Check sheet for the modelled part. Datum: model origin and axes. Units: mm. Face numbers are marked on the shaded views. Round coordinates to 2 decimals unless told otherwise and drop trailing zeros. Order: outer loops, then holes, each group sorted by start corner. A loop starts at its lowest first (then second) coordinate and runs counter-clockwise, first axis right, second up.
Q1. Cross-section at A-A on x = 7. Record the cut outline in (y, z).
Q2. Mould release check, pull along Y, two halves, no side actions. Record for the marked faces 1, 2 and 3: +Y half, -Y half, draft (parallel to the pull), parting line (faces both ways), or undercut.
Q3. Cross-section at C-C on z = -91.5. Record the cut outline in (x, y), then the cut area to 3 significant figures.
Q4. Depth check by flat-ended pin: P1, Ø4, axis at x = 100.5, y = 162, coming from the -Z side; P2, Ø11, axis at x = -104.5, y = 172, coming from the +Z side. Enter the tip coordinate at first touch or a pass-through.
Q5. Cross-section at B-B on y = 288.5. Record the cut outline in (x, z).
Q6. Cross-section at D-D on z = 0. Record the cut outline in (x, y), then the cut area to 3 significant figures.
Q7. Scan lines: probe 1 along Z at (x, y) = (154, 102.5); probe 2 along X at (y, z) = (159.5, 34); probe 3 along Y at (x, z) = (-168.5, -90.5). Record each from-to range of solid material in increasing order.
Autodesk Inventor part; units mm, degrees
ref_plane "YZ Plane" through (0, 0, 0) normal (1, 0, 0) x (0, 1, 0)
ref_plane "XZ Plane" through (0, 0, 0) normal (0, 1, 0) x (-1, 0, 0)
ref_plane "XY Plane" through (0, 0, 0) normal (0, 0, 1) x (1, 0, 0)
sketch "Boceto1" plane through (0, 0, 0) normal (0, 1, 0) x (-1, 0, 0)
  line L0 (200, 200) -> (-200, 200)
  line L1 (-200, 200) -> (-200, -200)
  line L2 (-200, -200) -> (200, -200)
  line L3 (200, -200) -> (200, 200)
  point P0 (0, 0)
  dimension "d0" = 400
  dimension "L" = 400
  dimension "d2" = 200
  dimension "d3" = 200
extrude "Extrusión1" add sketch "Boceto1" along normal blind 150
sketch "Boceto3" plane through (0, 150, 0) normal (0, 1, 0) x (1, 0, 0)
  circle A0 centre (0, -121) radius 39
  line L0 (200, 200) -> (-200, 200)
  line L1 (-200, -200) -> (200, -200)
  point P0 (0, 0)
  dimension "D" = 78
  dimension "d27" = 79
extrude "Extrusión2" [suppressed]
ref_plane "Plano de trabajo1" through (0, 0, 200) normal (1, 0, 0) x (0, 0, -1)
ref_plane "Plano de trabajo2" through (-200, 0, 0) normal (0, 0, 1) x (1, 0, 0)
sketch "Boceto4" plane through (0, 150, 0) normal (0, 1, 0) x (1, 0, 0)
  line L0 (-97.5, 140) -> (-97.5, -140)
  line L1 (97.5, 140) -> (97.5, -140)
  line L2 (200, 200) -> (-200, 200)
  circle A0 centre (0, -121) radius 39
  line L3 (-200, -200) -> (200, -200)
  line L4 (-97.5, -140) -> (-107.5, -140)
  line L5 (-107.5, -140) -> (-107.5, 140)
  line L6 (-107.5, 140) -> (-97.5, 140)
  line L7 (-97.5, 140) -> (-97.5, -140)
  line L8 (97.5, -140) -> (107.5, -140)
  line L9 (107.5, -140) -> (107.5, 140)
  line L10 (107.5, 140) -> (97.5, 140)
  line L11 (97.5, 140) -> (97.5, -140)
  point P0 (0, 0)
  dimension "Lriel" = 280
  dimension "d13" = 60
  dimension "d14" = 280
  dimension "d15" = 60
  dimension "d19" = 10
  dimension "d20" = 280
  dimension "d21" = 97.5
  dimension "d22" = 10
  dimension "d23" = 280
  dimension "d24" = 97.5
extrude "Extrusión3" add sketch "Boceto4" along normal blind 38 contours L0 L4 L5 L6 | L10 L9 L8 L1
sketch "Boceto5" plane through (0, 150, 0) normal (0, 1, 0) x (1, 0, 0)
  line L0 (-200, 200) -> (-200, -200)
  line L1 (-200, 200) -> (-200, 175)
  line L2 (-200, 175.482) -> (-195, 175.482)
  line L3 (-195, 175.482) -> (-195, 195.482)
  line L4 (-195, 195.482) -> (-175, 195.482)
  line L5 (-175, 195.482) -> (-175, 200)
  line L6 (200, 200) -> (-200, 200)
  line L7 (-200, 200) -> (-175, 200)
  line L8 (-200, -200) -> (-200, -175)
  line L9 (-200, -175) -> (-195, -175)
  line L10 (-195, -175) -> (-195, -195)
  line L11 (-195, -195) -> (-175, -195)
  line L12 (-175, -195) -> (-175, -200)
  line L13 (-200, -200) -> (200, -200)
  line L14 (-175, -200) -> (-200, -200)
  line L15 (200, -200) -> (200, 200)
  line L16 (200, -200) -> (200, -175)
  line L17 (200, -175) -> (195, -175)
  line L18 (195, -175) -> (195, -195)
  line L19 (195, -195) -> (175, -195)
  line L20 (175, -195) -> (175, -200)
  line L21 (200, -200) -> (175, -200)
  line L22 (200, 200) -> (200, 175)
  line L23 (200, 175) -> (195, 175)
  line L24 (195, 175) -> (195, 195)
  line L25 (195, 195) -> (175, 195)
  line L26 (175, 195) -> (175, 200)
  line L27 (200, 200) -> (175, 200)
  point P0 (0, 0)
  dimension "d28" = 25
  dimension "d29" = 5
  dimension "d30" = 20
  dimension "d31" = 20
  dimension "d32" = 25
  dimension "d33" = 5
  dimension "d34" = 20
  dimension "d35" = 20
  dimension "d36" = 25
  dimension "d37" = 5
  dimension "d38" = 20
  dimension "d39" = 20
  dimension "d40" = 25
  dimension "d41" = 5
  dimension "d42" = 20
  dimension "d43" = 20
extrude "Extrusión4" add sketch "Boceto5" along normal blind 200 contours L6 L5 L4 L3 L2 L0 | L6 L15 L23 L24 L25 L26 | L9 L10 L11 L12 L13 L0 | L15 L13 L20 L19 L18 L17
sketch "Boceto6" plane through (0, 350, 0) normal (0, 1, 0) x (1, 0, 0)
  line L0 (-200, 200) -> (-200, -200)
  line L1 (-200, -200) -> (200, -200)
  line L2 (200, -200) -> (200, 200)
  line L3 (200, 200) -> (-200, 200)
  line L4 (-200, 200) -> (-200, -200)
  point P0 (0, 0)
extrude "Extrusión5" add sketch "Boceto6" along normal blind 5
sketch "Boceto7" plane through (0, 150, 0) normal (0, 1, 0) x (1, 0, 0)
  line L0 (-200, 200) -> (-200, -200)
  line L1 (200, 200) -> (-200, 200)
  line L2 (200, -200) -> (200, 200)
  line L3 (-200, -200) -> (200, -200)
  circle A0 centre (154, 0) radius 39
  point P0 (0, 0)
  dimension "d48" = 78
  dimension "d49" = 200
  dimension "d50" = 46
extrude "Extrusión6" cut sketch "Boceto7" against normal blind 200.5 contours A0
sketch "Boceto8" plane through (107.5, 150, 140) normal (1, 0, 0) x (0, 0, -1)
  line L0 (61.75, 6.3333) -> (78.25, 6.3333) construction
  line L1 (61.75, 10.3333) -> (78.25, 10.3333)
  line L2 (78.25, 2.3333) -> (61.75, 2.3333)
  arc A0 (61.75, 10.3333) -> (61.75, 2.3333) centre (61.75, 6.3333) ccw
  arc A1 (78.25, 2.3333) -> (78.25, 10.3333) centre (78.25, 6.3333) ccw
  line L3 (0, 38) -> (280, 38)
  line L4 (0, 0) -> (0, 38)
  line L5 (198.75, 6.3333) -> (221.25, 6.3333) construction
  line L6 (315.482, 0) -> (-35, 0)
  line L7 (198.75, 10.3333) -> (221.25, 10.3333)
  line L8 (221.25, 2.3333) -> (198.75, 2.3333)
  arc A2 (198.75, 10.3333) -> (198.75, 2.3333) centre (198.75, 6.3333) ccw
  arc A3 (221.25, 2.3333) -> (221.25, 10.3333) centre (221.25, 6.3333) ccw
  line L9 (280, 0) -> (280, 38)
  point P0 (140, -150)
  point P1 (70, 6.3333)
  point P2 (210, 6.3333)
  dimension "d53" = 31.6667
  dimension "d54" = 70
  dimension "d55" = 4
  dimension "d56" = 31.6667
  dimension "d57" = 4
  dimension "d58" = 70
extrude "Extrusión7" cut sketch "Boceto8" against normal blind 251.25 contours L1 A1 L2 A0 | L7 A3 L8 A2
equation "\"d0\" = L"
equation "\"d14\" = Lriel"
properties part number "CajaBoya"
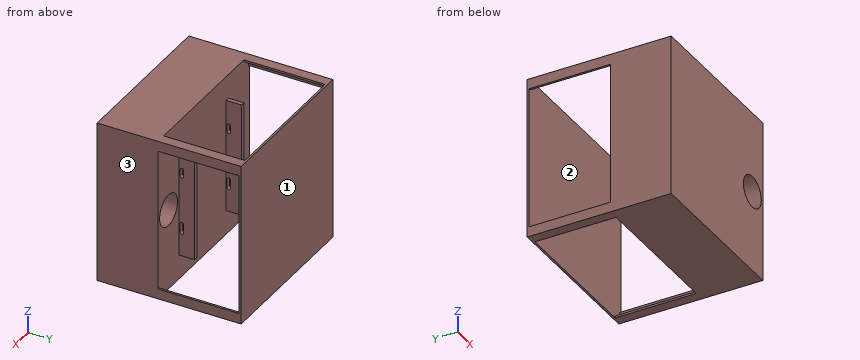
Results found:
1. outline: (0, -200) - (150, -200) - (150, 200) - (0, 200) - close; (350, -200) - (355, -200) - (355, 200) - (350, 200) - close
2. face 1: +Y half
2. face 2: undercut
2. face 3: draft
3. outline: (-200, 0) - (200, 0) - (200, 150) - (107.5, 150) - (107.5, 188) - (97.5, 188) - (97.5, 150) - (-97.5, 150) - (-97.5, 188) - (-107.5, 188) - (-107.5, 150) - (-200, 150) - close; (-200, 350) - (200, 350) - (200, 355) - (-200, 355) - close
3. area: 62,800 mm2
4. P1: stops at z = -140
4. P2: stops at z = 140
5. outline: (-200, -200) - (-175, -200) - (-175, -195.48) - (-195, -195.48) - (-195, -175.48) - (-200, -175.48) - close; (-200, 175) - (-195, 175) - (-195, 195) - (-175, 195) - (-175, 200) - (-200, 200) - close; (175, -200) - (200, -200) - (200, -175) - (195, -175) - (195, -195) - (175, -195) - close; (175, 195) - (195, 195) - (195, 175) - (200, 175) - (200, 200) - (175, 200) - close
6. outline: (-200, 0) - (115, 0) - (115, 150) - (107.5, 150) - (107.5, 188) - (97.5, 188) - (97.5, 150) - (-97.5, 150) - (-97.5, 188) - (-107.5, 188) - (-107.5, 150) - (-200, 150) - close; (-200, 350) - (200, 350) - (200, 355) - (-200, 355) - close; (193, 0) - (200, 0) - (200, 150) - (193, 150) - close
6. area: 51,100 mm2
7. probe 1: z = -200 to -39, 39 to 200
7. probe 2: x = -107.5 to -97.5, 97.5 to 107.5
7. probe 3: y = 0 to 150, 350 to 355
